CAD build for the part. Positions are in the model's coordinates, mm. A direction names the side the tool comes from. Round coordinates to 2 decimals unless told otherwise and drop trailing zeros. Write each loop counter-clockwise with the first axis right and the second up, starting at its lowest first coordinate (ties: lowest second). Pieces come first, ordered by that corner, then holes. Notation, with made-up numbers: (81, -2.5) - (126, -2.5) arc R29 ccw to (126, 21.5) - close; hole circle Ø2 at (17.25, -10.75). An arc over 180 degrees is marked (long way). Use one line per item in the form item = value. Start each with the question number.
Item 1: Band-saw the part on A-A, the plane x = 1. List the corners of the cut face in (y, z).
Item 2: Drill centre lines: L1, parallel to Y at x = 2.1, z = -43.5; L2, parallel to Y at x = 0.25, z = -35.5. Where is each one in solid material? Low to high.
Item 3: Tool access for faces 1 (the flat face through (1, 0, -63)), 2 (the flat face through (1, 18, 0)), 3 (the flat face through (1, 32, -16)), 4 (the flat face through (1, 0, -3)), 5 (the flat face through (1, -2, -26)): list every direction of +Z, -Z, +X, -X, +Y, -Y with a clear straight run to the whole face (end or side of a thin tool).
Item 4: Band-saw the part on B-B, the plane z = -8. List the corners of the cut face in (x, y), and give its area (3 significant figures).
Item 5: Pin check, flat tips, straight feed: pin 1 (1.5 mm diameter, centred on x = 1.5, y = 33.5, fed in from +Z); pin 2 (1.5 mm diameter, centred on x = 1.5, y = -1, fed in from -Z); pin 3 (0.9 mm diameter, centred on x = 1, y = -1, fed in from +Z); pin 4 (1.5 mm diameter, centred on x = 1, z = -47, fed in from +Y). Stop position of each tip, or through.
Item 6: Pull direction Z, two halves, no side cores. Call faces 6 (the flat face through (1, -1, -6)), 7 (the flat face through (1, 35, -34)), 8 (the flat face through (1, 34, -26)), 9 (the flat face through (1, -1, -41)): +Z half, -Z half, draft (parallel to the pull), parting line (faces both ways), or undercut.
from build123d import *

# Parameters (mm, degrees)
BOSS_EXTRUDE1_DEPTH = 3
SKETCH2_W           = 211.5
SKETCH2_H           = 45
CUT_EXTRUDE1_DEPTH  = 10


with BuildPart() as part:
    # Sketch1 → Boss-Extrude1 (new body)
    with BuildSketch(Plane(origin=(0, 0, 0), x_dir=(0, 0, -1), z_dir=(1, 0, 0))):
        Polygon((26, 0), (41, 0), (41, -3), (61, -3), (61, 0), (76, 0), (76, -3), (96, -3), (96, 0), (111, 0), (111, -3), (131, -3), (131, 0), (146, 0), (146, -3), (166, -3), (166, 0), (181, 0), (181, -3), (201, -3), (201, 0), (216, 0), (216, -3), (236, -3), (236, 0), (251, 0), (251, -3), (271, -3), (271, 0), (277, 0), (277, 35), (271, 35), (271, 32), (251, 32), (251, 35), (236, 35), (236, 32), (216, 32), (216, 35), (201, 35), (201, 32), (181, 32), (181, 35), (166, 35), (166, 32), (146, 32), (146, 35), (131, 35), (131, 32), (111, 32), (111, 35), (96, 35), (96, 32), (76, 32), (76, 35), (61, 35), (61, 32), (41, 32), (41, 35), (26, 35), (26, 32), (6, 32), (6, 35), (0, 35), (0, 0), (6, 0), (6, -3), (26, -3), align=None)
    extrude(amount=BOSS_EXTRUDE1_DEPTH)

    # Sketch2 → Cut-Extrude1 (cut)
    with BuildSketch(Plane(origin=(3, 0, 0), x_dir=(0, 0, -1), z_dir=(1, 0, 0))):
        with Locations((171.25, 17.5)):
            Rectangle(SKETCH2_W, SKETCH2_H)
    extrude(amount=-CUT_EXTRUDE1_DEPTH, mode=Mode.SUBTRACT)


solid = part.part
Determined:
q1.outline = (-3, -61) - (0, -61) - (0, -65.5) - (35, -65.5) - (35, -61) - (32, -61) - (32, -41) - (35, -41) - (35, -26) - (32, -26) - (32, -6) - (35, -6) - (35, 0) - (0, 0) - (0, -6) - (-3, -6) - (-3, -26) - (0, -26) - (0, -41) - (-3, -41) - close
q2.L1 = -3 to 32
q2.L2 = 0 to 35
q3.face_1 = -Z, +X, -X, -Y
q3.face_2 = +Z, +X, -X, +Y, -Y
q3.face_3 = +X, -X, +Y
q3.face_4 = +Z, +X, -X, -Y
q3.face_5 = +X, -X, -Y
q4.outline = (0, -3) - (3, -3) - (3, 32) - (0, 32) - close
q4.area = 105 mm²
q5.pin_1 = 0
q5.pin_2 = -61
q5.pin_3 = -6
q5.pin_4 = 32
q6.face_6 = +Z half
q6.face_7 = draft
q6.face_8 = undercut
q6.face_9 = undercut
